Design review of the part built by this model. Coordinates are the model's own, in mm. Face numbers are marked on the shaded views. A direction names the side the tool comes from. Give positions to 0.01 mm unless a question says otherwise; leave off trailing zeros. Loops run counter-clockwise (first coordinate to the right, second up) from the corner with the lowest first, then second, coordinate; pieces in that order, holes last. Notation, with made-up numbers: M 27.5,68.5 L 78.5,68.5 A33 ccw 78.5,107.5 Z; hole C 55,84.25 d3. An arc over 180 degrees is marked long. Use one line per item in the form item = value. Start each with the question number.
from build123d import *

# Parameters (mm, degrees)
BOSS_EXTRUDE1_DEPTH     = 6
CUT_EXTRUDE3_DEPTH      = 4.7
CUT_EXTRUDE4_DEPTH      = 21.471687766
CUT_EXTRUDE4_DEPTH_BACK = 21.471687766
SKETCH4_R               = 0.75
SKETCH6_R               = 0.75
CUT_EXTRUDE6_DEPTH      = 21.471687766
LPATTERN1_COUNT         = 3
LPATTERN1_PITCH         = 4
SCALE1_SCALE            = 1.02


with BuildPart() as part:
    # Sketch2 → Boss-Extrude1 (new body)
    with BuildSketch(Plane.XY):
        with BuildLine():
            Line((-6, 0), (-3.720572803, -15.718868867))
            ThreePointArc((-3.720572803, -15.718868867), (-5.969e-06, -19), (3.720571311, -15.71888071))
            Line((3.720571311, -15.71888071), (6, 0))
            ThreePointArc((6, 0), (0, 6), (-6, 0))
        make_face()
    extrude(amount=BOSS_EXTRUDE1_DEPTH)

    # Sketch3 → Cut-Extrude3 (cut)
    with BuildSketch(Plane.XY):
        with BuildLine():
            Line((-3.75, 0), (-2.25, -15))
            ThreePointArc((-2.25, -15), (0, -17.25), (2.25, -15))
            Line((2.25, -15), (3.75, 0))
            ThreePointArc((3.75, 0), (0, 3.75), (-3.75, 0))
        make_face()
    extrude(amount=CUT_EXTRUDE3_DEPTH, mode=Mode.SUBTRACT)

    # Sketch4 → Cut-Extrude4 (cut, two sides: drawn at the far end of the back side and taken through both)
    with BuildSketch(Plane(origin=(0, 0, 4.7), x_dir=(-1, 0, 0), z_dir=(0, 0, -1)).offset(-CUT_EXTRUDE4_DEPTH_BACK)):
        Circle(SKETCH4_R)
    extrude(amount=CUT_EXTRUDE4_DEPTH + CUT_EXTRUDE4_DEPTH_BACK, mode=Mode.SUBTRACT)

    # Sketch6 → Cut-Extrude6 (cut, symmetric)
    with BuildSketch(Plane(origin=(0, 0, 4.7), x_dir=(-1, 0, 0), z_dir=(0, 0, -1))):
        with Locations((0, -4.5)):
            Circle(SKETCH6_R)
    cut_extrude6 = extrude(amount=CUT_EXTRUDE6_DEPTH, both=True, mode=Mode.SUBTRACT)

    # LPattern1: Cut-Extrude6 ×3
    with Locations(*[(0, -i * LPATTERN1_PITCH, 0) for i in range(1, LPATTERN1_COUNT)]):
        add(cut_extrude6, mode=Mode.SUBTRACT)


with BuildPart() as part_1:
    # Scale1: scaled about (6e-08, -5.397561761, 3.434577722)
    add(part.part.scale(SCALE1_SCALE).moved(Location((-1e-09, 0.107951235, -0.068691554))))


solid = part_1.part
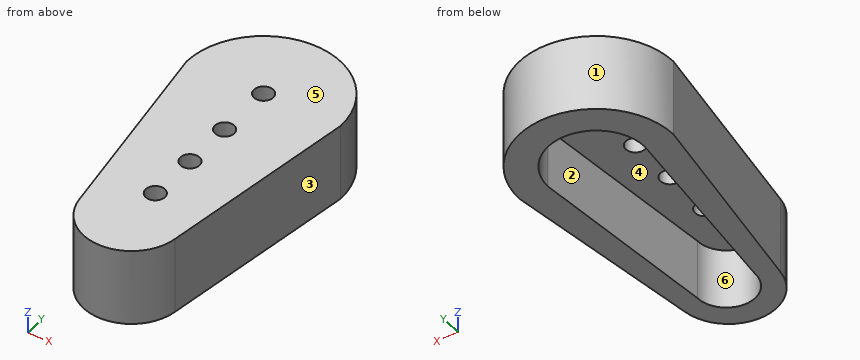
Q1. Take a section at A-A on x = 0. Give the boundary of the cut face in (y, z).
Q2. Take a section at B-B on y = 0.5. Give the boundary of the cut face in (x, z), plus the area to 3 significant figures.
Q3. Wall thickness on probe 1 along Y at (x, z) = (0, 5.6); probe 2 along Y at (x, z) = (0, 2); probe 3 along Z at (x, y) = (0.5, -10.5): over which ranges is each line inside the solid? List them lowest first.
Q4. Clearance check with flat-ended pins moving along their axes: pin 1 Ø1.4 at (x, y) = (0, 0.11) entering from -Z; pin 2 Ø2 at (y, z) = (-15, 2.5) entering from +X; pin 3 Ø1 at (y, z) = (-15.5, 4.5) entering from +X; pin 4 Ø1.8 at (x, y) = (0, -4.48) entering from -Z. State where each tip first meets the part, or that it passes through.
Q5. The part is to be moulded in two halves that separate along Y. For the marked faces 1, 2, 3 and 4, say which applies: pulls with the +Y half, pulls with the -Y half, needs draft (parallel to the pull), parting line crosses it, or undercut.
Q6. Take a section at C-C on z = 4.25. Give the boundary of the cut face in (x, y) (3 decimals), plus the area to 3 significant figures.
Q7. For the marked faces 5 and 6, list the 3-axis set-ups (+Z, -Z, +X, -X, +Y, -Y) from which the entire face can be reached by the end or side of a thin tool; tool diameter is ignored.
Q8. Take a section at D-D on z = 5.5. Give the boundary of the cut face in (x, y) (3 decimals), plus the area to 3 significant figures.
Response values:
q1.outline = M -19.27,-0.07 L -17.49,-0.07 L -17.49,4.73 L -13.41,4.73 L -13.41,6.05 L -19.27,6.05 Z; M -11.88,4.73 L -9.33,4.73 L -9.33,6.05 L -11.88,6.05 Z; M -7.8,4.73 L -5.25,4.73 L -5.25,6.05 L -7.8,6.05 Z; M -3.72,4.73 L -0.66,4.73 L -0.66,6.05 L -3.72,6.05 Z; M 0.87,4.73 L 3.93,4.73 L 3.93,-0.07 L 6.23,-0.07 L 6.23,6.05 L 0.87,6.05 Z
q2.outline = M -6.11,-0.07 L -3.8,-0.07 L -3.8,4.73 L -0.66,4.73 L -0.66,6.05 L -6.11,6.05 Z; M 0.66,4.73 L 3.8,4.73 L 3.8,-0.07 L 6.11,-0.07 L 6.11,6.05 L 0.66,6.05 Z
q2.area = 36.5 mm^2
q3.probe_1 = -19.27 to -13.41, -11.88 to -9.33, -7.8 to -5.25, -3.72 to -0.66, 0.87 to 6.23
q3.probe_2 = -19.27 to -17.49, 3.93 to 6.23
q3.probe_3 = 4.73 to 6.05
q4.pin_1 = through
q4.pin_2 = 4.07
q4.pin_3 = 3.93
q4.pin_4 = 4.73
q5.face_1 = pulls with the +Y half
q5.face_2 = undercut
q5.face_3 = pulls with the -Y half
q5.face_4 = undercut
q6.outline = M -6.12,0.108 L -3.795,-15.925 A3.825 ccw 3.795,-15.925 L 6.12,0.108 A6.12 ccw Z; hole M -3.825,0.108 L -2.295,-15.192 A2.295 ccw 2.295,-15.192 L 3.825,0.108 A3.825 ccw Z
q6.area = 112 mm^2
q7.face_5 = +Z, +X, -X, +Y, -Y
q7.face_6 = -Z
q8.outline = M -6.12,0.108 L -3.795,-15.925 A3.825 ccw 3.795,-15.925 L 6.12,0.108 A6.12 ccw Z; hole C 0,-12.642 d1.53; hole C 0,-8.562 d1.53; hole C 0,-4.482 d1.53; hole C 0,0.108 d1.53
q8.area = 230 mm^2
